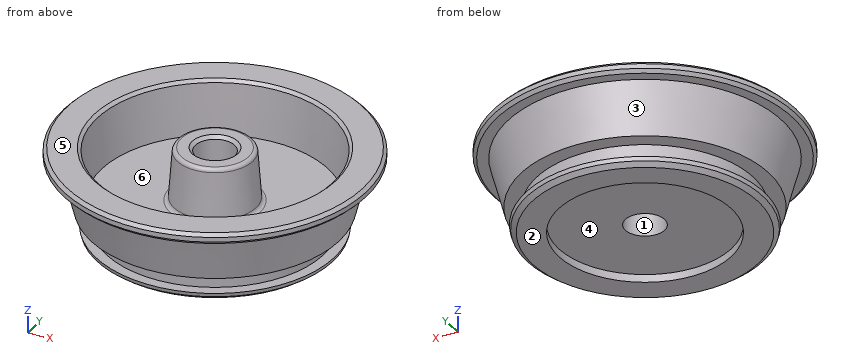
```python
from build123d import *

# Parameters (mm, degrees)
F3_R     = 0.5
F4_R     = 11
F5_DEPTH = 1
F6_SIZE  = 0.5


# Not quite as in the source:
# - a fillet or chamfer that OpenCascade refuses, or shapes differently, is made with other operations: its cross-section is extruded or revolved along the edge and cut away or added


with BuildPart() as f1:
    # F0 (on Front) → F1 (revolve)
    with BuildSketch(Plane.XZ):
        Polygon((4.75, 11), (2.5, 11), (2.5, 0), (14.8776877527, 0), (15.1418584287, 0.9858983849), (13.8, 0.9858983849), (13.8, 3.2858983849), (15.7581415713, 3.2858983849), (17.45, 9.6), (19.2, 9.6), (19.2, 11), (15, 11), (14.405077088, 4.2), (5.25, 4.2), align=None)
    revolve(axis=Axis((0, 0, 5.5), (0, 0, 1)))

    # F2: chamfer of 0.4 on 4 edges, made by hand

    # F2_s1 → F2_t2 (revolve, cut)
    with BuildSketch(Plane.XZ):
        Polygon((2.9, 11), (2.5, 10.6), (2.5, 11), align=None)
    revolve(axis=Axis((0, 0, 11), (0, 0, 1)), mode=Mode.SUBTRACT)

    # F2_s3 → F2_t4 (revolve, cut)
    with BuildSketch(Plane.XZ):
        Polygon((19.2, 10.6), (18.8, 11), (19.2, 11), align=None)
    revolve(axis=Axis((0, 0, 11), (0, 0, 1)), mode=Mode.SUBTRACT)

    # F2_s5 → F2_t6 (revolve, cut)
    with BuildSketch(Plane.XZ):
        Polygon((15.3665324696, 11), (14.9680545904, 10.6348622971), (15, 11), align=None)
    revolve(axis=Axis((0, 0, 11), (0, 0, 1)), mode=Mode.SUBTRACT)

    # F2_s7 → F2_t8 (revolve, cut)
    with BuildSketch(Plane.XZ):
        Polygon((18.8, 9.6), (19.2, 10), (19.2, 9.6), align=None)
    revolve(axis=Axis((0, 0, 9.6), (0, 0, 1)), mode=Mode.SUBTRACT)

    # F3
    f3_edges = [f1.edges().sort_by_distance(p)[0] for p in [
        (-5.25, 0, 4.2),
        (-4.75, 0, 11),
        (5, 0, 7.6),
    ]]
    fillet(f3_edges, radius=F3_R)

    # F4 (on face) → F5 (cut)
    with BuildSketch(Plane(origin=(0, 0, 0), x_dir=(1, 0, 0), z_dir=(0, 0, -1))):
        Circle(F4_R)
    extrude(amount=-F5_DEPTH, mode=Mode.SUBTRACT)

    # F6
    f6_edges = [f1.edges().sort_by_distance(p)[0] for p in [
        (-14.877688, 0, 0),
    ]]
    chamfer(f6_edges, length=F6_SIZE)


solid = f1.part
```
Part model, mm, in its own coordinate system. Face numbers are marked on the shaded views. A direction names the side the tool comes from. Round coordinates to 2 decimals unless told otherwise and drop trailing zeros. Loops run counter-clockwise (first coordinate to the right, second up) from the corner with the lowest first, then second, coordinate; pieces in that order, holes last. Notation, with made-up numbers: (74, 53.5) -> (120, 53.5) arc R15 ccw to (120, 59.5) -> close; hole circle Ø8 at (-20.5, 9.25). An arc over 180 degrees is marked (long way). Use CSV: the item, a comma, the result in double quotes. Start each with the question number.
1) Wall check: L1, parallel to Y at x = 0, z = 3; L2, parallel to Y at x = 0, z = 4.5; L3, parallel to Z at x = -7, y = -9.5. Give the ranges that are in metal, low to high. Write a range as [from, to].
2) Cut at A-A, the plane z = 7. Write the cut outline in (x, y).
3) Pull direction X, two halves, no side cores. Call the marked faces 1, 2 and 3: +X half, -X half, draft (parallel to the pull), parting line (faces both ways), or undercut.
4) Drop flat-ended pins along their axis: P1, Ø1, axis at y = 9, z = 5.5, coming from the +X side; P2, Ø5, axis at y = 12.5, z = 8, coming from the +X side; P3, Ø19, axis at x = 6.5, y = -8, coming from the -Z side; P4, Ø17.5, axis at x = 0, y = 0, coming from the -Z side. Give the stop position or say it passes through.
5) Which spindle directions (+Z, -Z, +X, -X, +Y, -Y) get a long thin tool onto all of the face, cutting with end or side? Do the marked faces 4, 5 and 6. Say none if no direction does.
6) Cut at B-B, the plane z = 2.5. Write the cut outline in (x, y), plus the area to 3 significant figures.
Determined:
1,L1,"y = [-13.8, -2.5], [2.5, 13.8]"
1,L2,"y = [-16.08, -14.43], [-5.26, -2.5], [2.5, 5.26], [14.43, 16.08]"
1,L3,"z = [0, 4.2]"
2,outline,"circle Ø33.51 at (0, 0); circle Ø10.09 at (0, 0); hole circle Ø29.3 at (0, 0); hole circle Ø5 at (0, 0)"
3,face 1,"undercut"
3,face 2,"draft"
3,face 3,"parting line"
4,P1,"stops at x = 14.01"
4,P2,"stops at x = 15.74"
4,P3,"stops at z = 0"
4,P4,"stops at z = 1"
5,face 4,"-Z"
5,face 5,"+Z, +X, -X, +Y, -Y"
5,face 6,"+Z"
6,outline,"circle Ø27.6 at (0, 0); hole circle Ø5 at (0, 0)"
6,area,"579 mm2"
